```python
from build123d import *

# Parameters (mm, degrees)
F1_DEPTH = 25.4
F2_SIZE  = 5.08
F3_R     = 5.08


with BuildPart() as f1:
    # F0 (on Top) → F1 (new body)
    with BuildSketch(Plane.XY):
        Polygon((19.4402, -9.906404), (19.4402, 22.270419), (-62.312644, 22.270419), (-62.312644, -9.906404), (-20.164922, -9.906404), align=None)
    extrude(amount=F1_DEPTH)

    # F2
    f2_edges = [f1.edges().sort_by_distance(p)[0] for p in [
        (19.4402, 22.270419, 12.7),
        (-62.312644, 22.270419, 12.7),
        (-21.436222, 22.270419, 0),
        (-21.436222, 22.270419, 25.4),
    ]]
    chamfer(f2_edges, length=F2_SIZE)

    # F3
    f3_edges = [f1.edges().sort_by_distance(p)[0] for p in [
        (-62.312644, -9.906404, 12.7),
        (-21.436222, -9.906404, 25.4),
        (19.4402, -9.906404, 12.7),
        (-21.436222, -9.906404, 0),
        (19.4402, 3.642007, 0),
        (-62.312644, 3.642007, 0),
    ]]
    fillet(f3_edges, radius=F3_R)


solid = f1.part
```
Part model, mm, in its own coordinate system. Round coordinates to 2 decimals unless told otherwise and drop trailing zeros. Loops run counter-clockwise (first coordinate to the right, second up) from the corner with the lowest first, then second, coordinate; pieces in that order, holes last. Notation, with made-up numbers: (36, 71.25) -> (55, 71.25) arc R13 ccw to (55, 80.25) -> close; hole circle Ø7 at (-39.75, -29.5). An arc over 180 degrees is marked (long way). Use a Markdown table: item, result.
1) Cut at A-A, the plane x = -56. List the corners of the cut face in (y, z), and give its area (3 significant figures).
The answers:
| item | result |
|---|---|
| outline | (-9.91, 5.08) arc R5.08 ccw to (-4.83, 0) -> (17.19, 0) -> (22.27, 5.08) -> (22.27, 20.32) -> (17.19, 25.4) -> (-4.83, 25.4) arc R5.08 ccw to (-9.91, 20.32) -> close |
| area | 780 mm2 |
2) Cut at B-B, the plane z = 23.5. List the corners of the cut face in (x, y), and give its area (3 significant figures).
The answers:
| item | result |
|---|---|
| outline | (-62.31, -4.83) arc R5.08 ccw to (-60.41, -8.79) -> (17.54, -8.79) arc R5.08 ccw to (19.44, -4.83) -> (19.44, 17.19) -> (17.54, 19.09) -> (-60.41, 19.09) -> (-62.31, 17.19) -> close |
| area | 2,270 mm2 |
3) Probe line 1 (X direction, y = -5, z = 8.5); line 2 (Z direction, x = -40, y = 20); line 3 (X direction, y = 0.5, z = 4.25). List the from-to ranges inside material, lowest first. Write a range as [from, to].
The answers:
| item | result |
|---|---|
| line 1 | x = [-62.31, 19.44] |
| line 2 | z = [2.81, 22.59] |
| line 3 | x = [-62.24, 19.37] |
